from build123d import *

# Parameters (mm, degrees)
ESQUISSE1_W             = 21.4234776
ESQUISSE1_H             = 23.749
BOSS_EXTRU_1_DEPTH      = 11.684
BOSS_EXTRU_2_DEPTH      = 4.318
BOSS_EXTRU_2_DEPTH_BACK = 28.067
ESQUISSE2_W             = 3.429
ESQUISSE2_H             = 11.684
ENL_V_MAT_EXTRU_1_REACH = 38.567
ESQUISSE4_R             = 1.016
CONG_1_R                = 1
ESQUISSE5_R             = 6.0198
BOSS_EXTRU_3_DEPTH      = 4.7244
ESQUISSE6_W             = 1
ESQUISSE6_H             = 23.749
ENL_V_MAT_EXTRU_2_DEPTH = 4.7244


with BuildPart() as part:
    # Esquisse1 → Boss.-Extru.1 (new body)
    with BuildSketch(Plane.XY):
        with Locations((10.7117388, 11.8745)):
            Rectangle(ESQUISSE1_W, ESQUISSE1_H)
    extrude(amount=BOSS_EXTRU_1_DEPTH)

    # Esquisse2 → Boss.-Extru.2 (add, two sides: drawn at the far end of the back side and taken through both)
    with BuildSketch(Plane.XZ.offset(-BOSS_EXTRU_2_DEPTH_BACK)):
        with Locations((2.8179776, 5.842)):
            Rectangle(ESQUISSE2_W, ESQUISSE2_H)
    extrude(amount=BOSS_EXTRU_2_DEPTH + BOSS_EXTRU_2_DEPTH_BACK)

    # Esquisse4 → Enlèv. mat.-Extru.1 (cut, up to next)
    with BuildSketch(Plane.ZY.offset(-1.1034776), mode=Mode.PRIVATE) as enl_v_mat_extru_1_sk1:
        with Locations((2.54, -1.778)):
            Circle(ESQUISSE4_R)
    enl_v_mat_extru_1_tool1 = extrude(enl_v_mat_extru_1_sk1.sketch, amount=-ENL_V_MAT_EXTRU_1_REACH, mode=Mode.PRIVATE) & part.part
    # Esquisse4 → Enlèv. mat.-Extru.1 (cut, up to next)
    with BuildSketch(Plane.ZY.offset(-1.1034776), mode=Mode.PRIVATE) as enl_v_mat_extru_1_sk2:
        with Locations((5.842, -2.286)):
            Circle(ESQUISSE4_R)
    enl_v_mat_extru_1_tool2 = extrude(enl_v_mat_extru_1_sk2.sketch, amount=-ENL_V_MAT_EXTRU_1_REACH, mode=Mode.PRIVATE) & part.part
    # Esquisse4 → Enlèv. mat.-Extru.1 (cut, up to next)
    with BuildSketch(Plane.ZY.offset(-1.1034776), mode=Mode.PRIVATE) as enl_v_mat_extru_1_sk3:
        with Locations((9.144, -1.778)):
            Circle(ESQUISSE4_R)
    enl_v_mat_extru_1_tool3 = extrude(enl_v_mat_extru_1_sk3.sketch, amount=-ENL_V_MAT_EXTRU_1_REACH, mode=Mode.PRIVATE) & part.part
    # Esquisse4 → Enlèv. mat.-Extru.1 (cut, up to next)
    with BuildSketch(Plane.ZY.offset(-1.1034776), mode=Mode.PRIVATE) as enl_v_mat_extru_1_sk4:
        with Locations(Location((9.144, 25.527, 0), (0, 0, 180))):
            Circle(ESQUISSE4_R)
    enl_v_mat_extru_1_tool4 = extrude(enl_v_mat_extru_1_sk4.sketch, amount=-ENL_V_MAT_EXTRU_1_REACH, mode=Mode.PRIVATE) & part.part
    # Esquisse4 → Enlèv. mat.-Extru.1 (cut, up to next)
    with BuildSketch(Plane.ZY.offset(-1.1034776), mode=Mode.PRIVATE) as enl_v_mat_extru_1_sk5:
        with Locations(Location((5.842, 26.035, 0), (0, 0, 180))):
            Circle(ESQUISSE4_R)
    enl_v_mat_extru_1_tool5 = extrude(enl_v_mat_extru_1_sk5.sketch, amount=-ENL_V_MAT_EXTRU_1_REACH, mode=Mode.PRIVATE) & part.part
    # Esquisse4 → Enlèv. mat.-Extru.1 (cut, up to next)
    with BuildSketch(Plane.ZY.offset(-1.1034776), mode=Mode.PRIVATE) as enl_v_mat_extru_1_sk6:
        with Locations(Location((2.54, 25.527, 0), (0, 0, 180))):
            Circle(ESQUISSE4_R)
    enl_v_mat_extru_1_tool6 = extrude(enl_v_mat_extru_1_sk6.sketch, amount=-ENL_V_MAT_EXTRU_1_REACH, mode=Mode.PRIVATE) & part.part
    add(enl_v_mat_extru_1_tool1.solids().sort_by_distance((1.103478, -1.778, 2.54))[0], mode=Mode.SUBTRACT)
    add(enl_v_mat_extru_1_tool2.solids().sort_by_distance((1.103478, -2.286, 5.842))[0], mode=Mode.SUBTRACT)
    add(enl_v_mat_extru_1_tool3.solids().sort_by_distance((1.103478, -1.778, 9.144))[0], mode=Mode.SUBTRACT)
    add(enl_v_mat_extru_1_tool4.solids().sort_by_distance((1.103478, 25.527, 9.144))[0], mode=Mode.SUBTRACT)
    add(enl_v_mat_extru_1_tool5.solids().sort_by_distance((1.103478, 26.035, 5.842))[0], mode=Mode.SUBTRACT)
    add(enl_v_mat_extru_1_tool6.solids().sort_by_distance((1.103478, 25.527, 2.54))[0], mode=Mode.SUBTRACT)

    # Congé1
    cong_1_edges = [part.edges().sort_by_distance(p)[0] for p in [
        (2.8179776, 28.067, 11.684),
        (2.8179776, 28.067, 0),
        (2.8179776, -4.318, 0),
        (2.8179776, -4.318, 11.684),
    ]]
    fillet(cong_1_edges, radius=CONG_1_R)

    # Esquisse5 → Boss.-Extru.3 (add)
    with BuildSketch(Plane.ZY):
        with Locations(Location((5.864615101, 17.7292, 0), (0, 0, 166.962066999))):
            Circle(ESQUISSE5_R)
    extrude(amount=BOSS_EXTRU_3_DEPTH)

    # Esquisse6 → Enlèv. mat.-Extru.2 (cut)
    with BuildSketch(Plane.ZY):
        with Locations((12.184, 11.8745)):
            Rectangle(ESQUISSE6_W, ESQUISSE6_H)
        with Locations((-0.5, 11.8745)):
            Rectangle(ESQUISSE6_W, ESQUISSE6_H)
    extrude(amount=ENL_V_MAT_EXTRU_2_DEPTH, mode=Mode.SUBTRACT)


solid = part.part
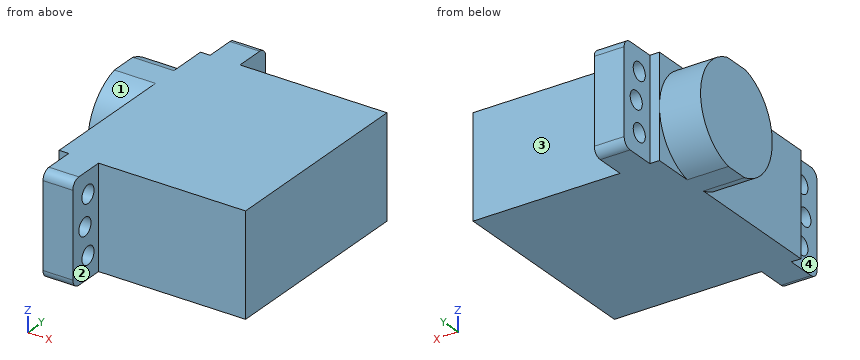
Read the model definition and answer for the solid it produces. Units are mm, in the model's axes. Face numbers are marked on the shaded views. A direction names the side the tool comes from. Coordinates: 2 decimals unless noted, no trailing zeros. Write each loop counter-clockwise with the first axis right and the second up, starting at its lowest first coordinate (ties: lowest second). Pieces come first, ordered by that corner, then holes. Notation, with made-up numbers: M 22.5,60.5 L 40.5,60.5 A19 ccw 40.5,78.5 Z; hole C 66,26.25 d7. An arc over 180 degrees is marked long. Use a Markdown table: item, result.
Q1. The part is cut by section A-A, the plane z = 8.5. Write down the section's boundary in (x, y), then the cut area to 3 significant figures.
Answer block:
| item | result |
|---|---|
| outline | M -4.72,12.32 L 0,12.32 L 0,0 L 1.1,0 L 1.1,-0.99 L 4.53,-0.99 L 4.53,0 L 21.42,0 L 21.42,23.75 L 4.53,23.75 L 4.53,24.74 L 1.1,24.74 L 1.1,23.75 L 0,23.75 L 0,23.14 L -4.72,23.14 Z; M 1.1,-4.32 L 4.53,-4.32 L 4.53,-2.56 L 1.1,-2.56 Z; M 1.1,26.31 L 4.53,26.31 L 4.53,28.07 L 1.1,28.07 Z |
| area | 579 mm2 |
Q2. Straight lines are drawn through the part: L1, parallel to Y at x = 3.1, z = 2.54; L2, parallel to X at y = 1, z = 1.5; L3, parallel to Y at x = 20.25, z = 6. For each, find the intervals that lie inside material, in ascending order. Write a range as [from, to].
Answer block:
| item | result |
|---|---|
| L1 | y = [-4.32, -2.79], [-0.76, 24.51], [26.54, 28.07] |
| L2 | x = [0, 21.42] |
| L3 | y = [0, 23.75] |
Q3. The part is cut by section C-C, the plane y = 22. Write down the section's boundary in (x, z).
Answer block:
| item | result |
|---|---|
| outline | M -4.72,1.62 L 0,1.62 L 0,0 L 21.42,0 L 21.42,11.68 L 0,11.68 L 0,10.11 L -4.72,10.11 Z |
Q4. The part is cut by section D-D, the plane z = 2.5. Write down the section's boundary in (x, y).
Answer block:
| item | result |
|---|---|
| outline | M -4.72,12.74 L 0,12.74 L 0,0 L 1.1,0 L 1.1,-0.76 L 4.53,-0.76 L 4.53,0 L 21.42,0 L 21.42,23.75 L 4.53,23.75 L 4.53,24.51 L 1.1,24.51 L 1.1,23.75 L 0,23.75 L 0,22.72 L -4.72,22.72 Z; M 1.1,-4.32 L 4.53,-4.32 L 4.53,-2.79 L 1.1,-2.79 Z; M 1.1,26.54 L 4.53,26.54 L 4.53,28.07 L 1.1,28.07 Z |
Q5. Each of these flat-tipped pins is pushed along its axis until it touches: pin 1 Ø3.5 at (y, z) = (-2.286, 5.842) entering from -X; pin 2 Ø1.3 at (y, z) = (26, 4) entering from +X; pin 3 Ø0.6 at (x, z) = (0.5, 8.5) entering from -Y. Where does it stop, or does it pass through?
Answer block:
| item | result |
|---|---|
| pin 1 | stops at x = 1.1 |
| pin 2 | stops at x = 4.53 |
| pin 3 | stops at y = 0 |
Q6. Which of the six approach directions +Z, -Z, +X, -X, +Y, -Y give full straight-line access (tool end or side, diameter ignored) to the marked faces 1, 2, 3 and 4?
Answer block:
| item | result |
|---|---|
| face 1 | -X, -Y |
| face 2 | +Z, -Z, +X, -Y |
| face 3 | +Z, -Z, +X, +Y |
| face 4 | +Z, -Z, -X, -Y |
Q7. The part is cut by section B-B, the plane x = 4. Write down the section's boundary in (y, z) (3 decimals), then the cut area to 3 significant figures.
Answer block:
| item | result |
|---|---|
| outline | M -4.318,1 A1 ccw -3.318,0 L 27.067,0 A1 ccw 28.067,1 L 28.067,10.684 A1 ccw 27.067,11.684 L -3.318,11.684 A1 ccw -4.318,10.684 Z; hole C -2.286,5.842 d2.032; hole C -1.778,2.54 d2.032; hole C -1.778,9.144 d2.032; hole C 25.527,2.54 d2.032; hole C 25.527,9.144 d2.032; hole C 26.035,5.842 d2.032 |
| area | 358 mm2 |
